Geometry check sheet. Reference: the model listing, model coordinates, mm. Round coordinates to 2 decimals unless told otherwise and drop trailing zeros. Write each loop counter-clockwise with the first axis right and the second up, starting at its lowest first coordinate (ties: lowest second). Pieces come first, ordered by that corner, then holes. Notation, with made-up numbers: (31, 17.25) - (84, 17.25) arc R9 ccw to (84, 28.25) - close; hole circle Ø2 at (82.25, -30). An arc over 180 degrees is marked (long way). One line per question, with ' | ' between items. Start each with the question number.
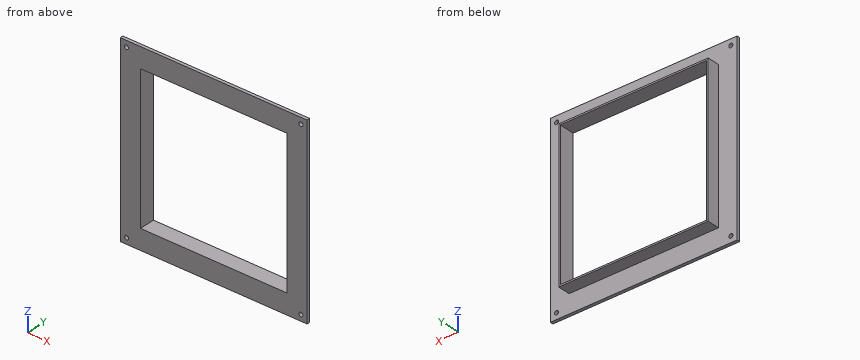
from build123d import *

# Parameters (mm, degrees)
BOSS_EXTRUDE1_DEPTH   = 5
SKETCH4_W             = 240
SKETCH4_H             = 240
SKETCH4_W_2           = 230.5
SKETCH4_H_2           = 230.5
BOSS_EXTRUDE2_DEPTH   = 20
SKETCH6_R             = 3.25
CUT_EXTRUDE1_DEPTH    = 20
SKETCH7_W             = 240
SKETCH7_H             = 240
CUT_EXTRUDE2_DEPTH    = 20
SKETCH8_W             = 240
SKETCH8_H             = 240
SKETCH8_W_2           = 235
SKETCH8_H_2           = 235
BOSS_EXTRUDE3_DEPTH   = 20
SKETCH9_W             = 235
SKETCH9_H             = 235
CUT_EXTRUDE3_DEPTH    = 20
BODY_MOVE_COPY1_ANGLE = 89.5
BODY_MOVE_COPY2_ANGLE = 90


with BuildPart() as part:
    # Sketch3 → Boss-Extrude1 (new body)
    with BuildSketch(Plane(origin=(0, 0, 0), x_dir=(1, 0, 0), z_dir=(0, 1, 0))):
        Polygon((300, 300), (150, 150), (300, 0), align=None)
        Polygon((150, 150), (0, 0), (300, 0), align=None)
        Polygon((0, 300), (0, 0), (150, 150), align=None)
        Polygon((0, 300), (150, 150), (300, 300), align=None)
    extrude(amount=BOSS_EXTRUDE1_DEPTH)

    # Sketch4 → Boss-Extrude2 (add)
    with BuildSketch(Plane(origin=(0, 5, 0), x_dir=(1, 0, 0), z_dir=(0, 1, 0))):
        with Locations((150, 150)):
            Rectangle(SKETCH4_W, SKETCH4_H)
        with Locations((150, 150)):
            Rectangle(SKETCH4_W_2, SKETCH4_H_2, mode=Mode.SUBTRACT)
    extrude(amount=BOSS_EXTRUDE2_DEPTH)

    # Sketch6 → Cut-Extrude1 (cut)
    with BuildSketch(Plane(origin=(0, 5, 0), x_dir=(1, 0, 0), z_dir=(0, 1, 0))):
        with Locations(Location((10, 10, 0), (0, 0, 270))):
            Circle(SKETCH6_R)
        with Locations(Location((290, 10, 0), (0, 0, 270))):
            Circle(SKETCH6_R)
        with Locations(Location((290, 290, 0), (0, 0, 270))):
            Circle(SKETCH6_R)
        with Locations(Location((10, 290, 0), (0, 0, 270))):
            Circle(SKETCH6_R)
    extrude(amount=-CUT_EXTRUDE1_DEPTH, mode=Mode.SUBTRACT)

    # Sketch7 → Cut-Extrude2 (cut)
    with BuildSketch(Plane(origin=(0, 25, 0), x_dir=(1, 0, 0), z_dir=(0, 1, 0))):
        with Locations((150, 150)):
            Rectangle(SKETCH7_W, SKETCH7_H)
    extrude(amount=-CUT_EXTRUDE2_DEPTH, mode=Mode.SUBTRACT)

    # Sketch8 → Boss-Extrude3 (add)
    with BuildSketch(Plane(origin=(0, 5, 0), x_dir=(1, 0, 0), z_dir=(0, 1, 0))):
        with Locations((150, 150)):
            Rectangle(SKETCH8_W, SKETCH8_H)
        with Locations((150, 150)):
            Rectangle(SKETCH8_W_2, SKETCH8_H_2, mode=Mode.SUBTRACT)
    extrude(amount=BOSS_EXTRUDE3_DEPTH)

    # Sketch9 → Cut-Extrude3 (cut)
    with BuildSketch(Plane(origin=(0, 5, 0), x_dir=(1, 0, 0), z_dir=(0, 1, 0))):
        with Locations((150, 150)):
            Rectangle(SKETCH9_W, SKETCH9_H)
    extrude(amount=-CUT_EXTRUDE3_DEPTH, mode=Mode.SUBTRACT)


with BuildPart() as part_1:
    # Body-Move/Copy1: moved
    add(part.part.rotate(Axis((150, 12.5, 0), (0, 0, -1)), BODY_MOVE_COPY1_ANGLE))


with BuildPart() as part_2:
    # Body-Move/Copy2: moved
    add(part_1.part.rotate(Axis((149.869101968, 12.412734645, 0), (0, 0, 1)), BODY_MOVE_COPY2_ANGLE))


solid = part_2.part
Q1. Thickness scan on line 1 (X direction, y = 6.5, z = -143.5); line 2 (X direction, y = 18.5, z = -142.5); line 3 (Z direction, x = 33.5, y = 22.5). Record the ranges inside material, lowest first.
Q2. Section check A-A, the plane z = -252. Record the cut outline in (x, y).
Q3. Section check C-C, the plane x = 173.5. Record the cut outline in (y, z), then the cut area to 3 significant figures.
Q4. Go/stop test with flat-tipped pins: P1, Ø6.5, axis at x = 102, y = 17.5, coming from the -Z side; P2, Ø2, axis at y = 20.5, z = -64, coming from the -X side; P3, Ø8, axis at y = 8.5, z = -173, coming from the -X side. Record where each tip stops, or that it passes through.
Q5. Section check B-B, the plane y = 15.75. Record the cut outline in (x, z), then the cut area to 3 significant figures.
Result sheet:
1) line 1: 29.83 to 32.33, 267.34 to 269.84 | line 2: 29.73 to 32.23, 267.23 to 269.73 | line 3: -270 to -267.5, -32.5 to -30
2) outline: (-0.15, 3.73) - (-0.1, -1.26) - (32.4, -0.98) - (32.18, 24.02) - (29.68, 24) - (29.85, 4) - close; (267.17, 26.07) - (267.39, 1.07) - (299.89, 1.35) - (299.84, 6.35) - (269.84, 6.09) - (269.67, 26.09) - close
3) outline: (0.25, -300) - (5.25, -300) - (5.25, -270) - (25.25, -270) - (25.25, -267.5) - (0.25, -267.5) - close; (0.25, -32.5) - (25.25, -32.5) - (25.25, -30) - (5.25, -30) - (5.25, 0) - (0.25, 0) - close | area: 425 mm²
4) P1: z = -270 | P2: x = 29.7 | P3: x = 29.78
5) outline: (29.75, -270) - (269.76, -270) - (269.76, -30) - (29.75, -30) - close; hole (32.25, -267.5) - (267.26, -267.5) - (267.26, -32.5) - (32.25, -32.5) - close | area: 2,380 mm²
